from build123d import *

# Parameters (mm, degrees)
SKETCH10_R                  = 2.5
BOSS_EXTRUDE1_DEPTH         = 37
BOSS_EXTRUDE2_START         = -10
SKETCH11_W                  = 25
SKETCH11_H                  = 25
BOSS_EXTRUDE2_DEPTH         = 30
SKETCH13_W                  = 20
SKETCH13_H                  = 15
CUT_EXTRUDE3_DEPTH          = 30
FILLET1_R                   = 1
M6_TAPPED_HOLE1_D           = 5
M6_TAPPED_HOLE1_DEPTH       = 30
M6_TAPPED_HOLE1_CSINK_D     = 6.05
M6_TAPPED_HOLE1_CSINK_ANGLE = 90
M6_TAPPED_HOLE1_TIP         = 1.502151548
M6_TAPPED_HOLE2_D           = 5
M6_TAPPED_HOLE2_DEPTH       = 30
M6_TAPPED_HOLE2_CSINK_D     = 6.05
M6_TAPPED_HOLE2_CSINK_ANGLE = 90
M6_TAPPED_HOLE2_TIP         = 1.502151548
SKETCH9_W                   = 18
SKETCH9_H                   = 4
CUT_EXTRUDE2_DEPTH          = 2
SKETCH14_R                  = 2.5
BOSS_EXTRUDE3_DEPTH         = 37.7
FILLET2_R                   = 1
SKETCH16_R                  = 4.5
BOSS_EXTRUDE4_DEPTH         = 1
SKETCH18_R                  = 4.5
BOSS_EXTRUDE6_DEPTH         = 1
BOSS_EXTRUDE7_DEPTH         = 5
BOSS_EXTRUDE7_DEPTH_BACK    = 30
SKETCH19_R                  = 2.5
FILLET3_R                   = 1


with BuildPart() as part:
    # Sketch2 → Revolve1 (revolve)
    with BuildSketch(Plane.XY, mode=Mode.PRIVATE) as revolve1_sk:
        Polygon((0, 0), (0, 17.5), (10, 17.5), (10, 15), (70, 15), (70, 17.5), (80, 17.5), (80, 15), (100, 15), (100, 5), (101, 5), (101, 2.5), (101, 0), (70.994843836, 0), align=None)
    revolve(revolve1_sk.sketch.rotate(Axis((0, 0, 0), (1, 0, 0)), 90), axis=Axis((0, 0, 0), (1, 0, 0)))

    # Sketch10 → Boss-Extrude1 (add)
    with BuildSketch(Plane(origin=(101, 0, 0), x_dir=(0, 0, -1), z_dir=(1, 0, 0))):
        with Locations(Location((0, 0, 0), (0, 0, 90))):
            Circle(SKETCH10_R)
    extrude(amount=BOSS_EXTRUDE1_DEPTH)

    # Sketch11 → Boss-Extrude2 (add)
    with BuildSketch(Plane(origin=(138, 0, 0), x_dir=(0, 0, -1), z_dir=(1, 0, 0)).offset(BOSS_EXTRUDE2_START)):
        Rectangle(SKETCH11_W, SKETCH11_H)
    extrude(amount=BOSS_EXTRUDE2_DEPTH)

    # Sketch13 → Cut-Extrude3 (cut)
    with BuildSketch(Plane(origin=(0, 12.5, 0), x_dir=(1, 0, 0), z_dir=(0, 1, 0))):
        with Locations((143, 0)):
            Rectangle(SKETCH13_W, SKETCH13_H)
    extrude(amount=-CUT_EXTRUDE3_DEPTH, mode=Mode.SUBTRACT)

    # Fillet1
    fillet1_edges = [part.edges().sort_by_distance(p)[0] for p in [
        (101, -2.5, 0),
        (128, -2.5, 0),
    ]]
    fillet(fillet1_edges, radius=FILLET1_R)

    # M6 Tapped Hole1
    with Locations(Plane(origin=(0, 0, 0), x_dir=(0, 0, -1), z_dir=(-1, 0, 0))):
        with Locations((0, 0)):
            CounterSinkHole(M6_TAPPED_HOLE1_D / 2, M6_TAPPED_HOLE1_CSINK_D / 2, depth=M6_TAPPED_HOLE1_DEPTH, counter_sink_angle=M6_TAPPED_HOLE1_CSINK_ANGLE)
            with Locations((0, 0, -(M6_TAPPED_HOLE1_DEPTH + M6_TAPPED_HOLE1_TIP / 2))):  # 118° drill point
                Cone(0, M6_TAPPED_HOLE1_D / 2, M6_TAPPED_HOLE1_TIP, mode=Mode.SUBTRACT)

    # M6 Tapped Hole2
    with Locations(Plane(origin=(0, -0.192029445, 8.997951139), x_dir=(0, 0, -1), z_dir=(-1, 0, 0))):
        with Locations((0, 0), (17.997918621, -0.167835984)):
            CounterSinkHole(M6_TAPPED_HOLE2_D / 2, M6_TAPPED_HOLE2_CSINK_D / 2, depth=M6_TAPPED_HOLE2_DEPTH, counter_sink_angle=M6_TAPPED_HOLE2_CSINK_ANGLE)
            with Locations((0, 0, -(M6_TAPPED_HOLE2_DEPTH + M6_TAPPED_HOLE2_TIP / 2))):  # 118° drill point
                Cone(0, M6_TAPPED_HOLE2_D / 2, M6_TAPPED_HOLE2_TIP, mode=Mode.SUBTRACT)

    # Sketch9 → Cut-Extrude2 (cut)
    with BuildSketch(Plane.ZY):
        Rectangle(SKETCH9_W, SKETCH9_H)
    extrude(amount=-CUT_EXTRUDE2_DEPTH, mode=Mode.SUBTRACT)

    # Sketch14 → Boss-Extrude3 (add)
    with BuildSketch(Plane(origin=(101, 0, 0), x_dir=(0, 0, -1), z_dir=(1, 0, 0))):
        with Locations(Location((0, 0, 0), (0, 0, 180))):
            Circle(SKETCH14_R)
    extrude(amount=BOSS_EXTRUDE3_DEPTH)

    # Fillet2
    fillet2_edges = [part.edges().sort_by_distance(p)[0] for p in [
        (138.7, 0, -2.5),
    ]]
    fillet(fillet2_edges, radius=FILLET2_R)

    # Sketch16 → Boss-Extrude4 (add)
    with BuildSketch(Plane(origin=(133, 0, 0), x_dir=(0, 0, -1), z_dir=(1, 0, 0))):
        with Locations(Location((0, 0, 0), (0, 0, 270))):
            Circle(SKETCH16_R)
    extrude(amount=BOSS_EXTRUDE4_DEPTH)

    # Sketch18 → Boss-Extrude6 (add)
    with BuildSketch(Plane.XY.offset(-7.5)):
        with Locations(Location((143, 0, 0), (0, 0, 180))):
            Circle(SKETCH18_R)
    extrude(amount=BOSS_EXTRUDE6_DEPTH)

    # Sketch19 → Boss-Extrude7 (add, two sides: drawn at the far end of the back side and taken through both)
    with BuildSketch(Plane.XY.offset(-6.5).offset(-BOSS_EXTRUDE7_DEPTH_BACK)):
        with Locations((143, 0)):
            Circle(SKETCH19_R)
    extrude(amount=BOSS_EXTRUDE7_DEPTH + BOSS_EXTRUDE7_DEPTH_BACK)

    # Fillet3
    fillet3_edges = [part.edges().sort_by_distance(p)[0] for p in [
        (140.5, 0, -1.5),
    ]]
    fillet(fillet3_edges, radius=FILLET3_R)


solid = part.part
Input: part model. Units: mm. Frame: model coordinates. A direction names the side the tool comes from. Coordinates: 2 decimals unless noted, no trailing zeros. Write each loop counter-clockwise with the first axis right and the second up, starting at its lowest first coordinate (ties: lowest second). Pieces come first, ordered by that corner, then holes. Notation, with made-up numbers: M 51.5,-9 L 95.5,-9 A13 cw 95.5,6 Z; hole C 64,19.5 d5. An arc over 180 degrees is marked long. Answer as a JSON object with one key per item and string values. Group by question number.
(1) Mould query, pull axis Z, two halves, no side actions, for faces 1 (the face through (5.07, 17.084, -3.794)), 2 (the face through (143, 0, -36.5)), 3 (the face through (133.493, -4.292, -1.352)). Classes: pulls with the +Z half, pulls with the -Z half, needs draft (parallel to the pull), parting line crosses it, or undercut.
(2) Section B-B on x = 103.5. Output: boundary loops of the cut face in (y, z).
(3) Set-up query: faces 4 (the face through (143, 0, 7.5)), 5 (the face through (2, 0, -5)), 6 (the face through (10, -8, 13)). Return all of +Z, -Z, +X, -X, +Y, -Y with unobstructed straight access to the full face (end or side cutting, diameter ignored); none if empty.
(4) Section A-A on x = 143. Output: boundary loops of the cut face in (y, z).
(5) Contact query for flat-ended pins moving along their axis: P1, Ø1.6, axis at x = 1.5, z = -5.5, coming from the +Y side; P2, Ø2, axis at y = 0.5, z = 4, coming from the -X side; P3, Ø5, axis at x = 35, y = 3.5, coming from the -Z side. Output: stop coordinate, or through.
(6) Section C-C on z = -21. Output: boundary loops of the cut face in (x, y).
(7) Ray query, line 1 along Y through (x, z) = (12.25, 0); line 2 along X through (y, z) = (-14.5, -7); line 3 along X through (y, z) = (-1, -6). Return the intervals inside material, ascending. Write a range as [from, to].
(8) Section D-D on x = 28. Output: boundary loops of the cut face in (y, z).
Result set:
{
 "1": {"face 1": "parting line crosses it", "face 2": "pulls with the -Z half", "face 3": "undercut"},
 "2": {"outline": "C 0,0 d5"},
 "3": {"face 4": "+Y, -Y", "face 5": "-X", "face 6": "none"},
 "4": {"outline": "M -12.5,-12.5 L -2.5,-12.5 L -2.5,-36.5 L 2.5,-36.5 L 2.5,-12.5 L 12.5,-12.5 L 12.5,-7.5 L 4.5,-7.5 L 4.5,-6.5 L 2.5,-6.5 L 2.5,-2.5 A1 ccw 1.5,-1.5 L -1.5,-1.5 A1 ccw -2.5,-2.5 L -2.5,-6.5 L -4.5,-6.5 L -4.5,-7.5 L -12.5,-7.5 Z; M -12.5,7.5 L 12.5,7.5 L 12.5,12.5 L -12.5,12.5 Z"},
 "5": {"P1": "stops at y = 16.86", "P2": "stops at x = 2", "P3": "stops at z = -14.97"},
 "6": {"outline": "C 143,0 d5"},
 "7": {"line 1": "y = [-15, -2.5], [2.5, 15]", "line 2": "x = [0, 10], [70, 80]", "line 3": "x = [2, 100], [128, 133], [140.71, 145.29], [153, 158]"},
 "8": {"outline": "C 0,0 d30; hole C -0.19,9 d5; hole C -0.02,-9 d5; hole C 0,0 d5"}
}
